Job drawing, mm, ordinate dimensions from the low corner. One solid piece. A direction names the side the tool comes from. Give positions to 0.01 mm unless a question says otherwise; leave off trailing zeros. Loops run counter-clockwise (first coordinate to the right, second up) from the corner with the lowest first, then second, coordinate; pieces in that order, holes last. Notation, with made-up numbers: (29, 28) -> (54, 28) arc R32 cw to (54, 60) -> close; hole circle Ø8 at (27.25, 3). An arc over 180 degrees is marked (long way). Answer as a JSON object with one key per item and string values. Group by question number.
Q1. Wall check: probe 1 along Z at (x, y) = (4, 3.3); probe 2 along X at (y, z) = (3.3, 3.5); probe 3 along Y at (x, z) = (6.5, 0.75) (3 decimals). Give the ranges that are in metal, low to high. Write a range as from..to.
Q2. Band-saw the part on C-C, the plane x = 1.25. Write the cut outline in (y, z) (3 decimals).
Q3. Drop flat-ended pins along their axis: pin 1 (1.2 mm diameter, centred on x = 3.5, z = 3.5, fed in from -Y); pin 2 (2 mm diameter, centred on y = 1, z = 4.5, fed in from +X). Give the stop position or say it passes through.
Q4. Band-saw the part on D-D, the plane z = 1. Write the cut outline in (x, y) (3 decimals).
Q5. Tool access for the marked faces 4, 5 and 6: list every direction of +Z, -Z, +X, -X, +Y, -Y with a clear straight run to the whole face (end or side of a thin tool).
Q6. Two-plate mould, pull along Z, no slides. Class the marked faces 1, 2 and 3: pulls with the +Z half, pulls with the -Z half, needs draft (parallel to the pull), parting line crosses it, or undercut.
Q7. Band-saw the part on B-B, the plane y = 2.5. Write the cut outline in (x, z).
Q8. Band-saw the part on A-A, the plane z = 4. Write the cut outline in (x, y) (1 decimal).
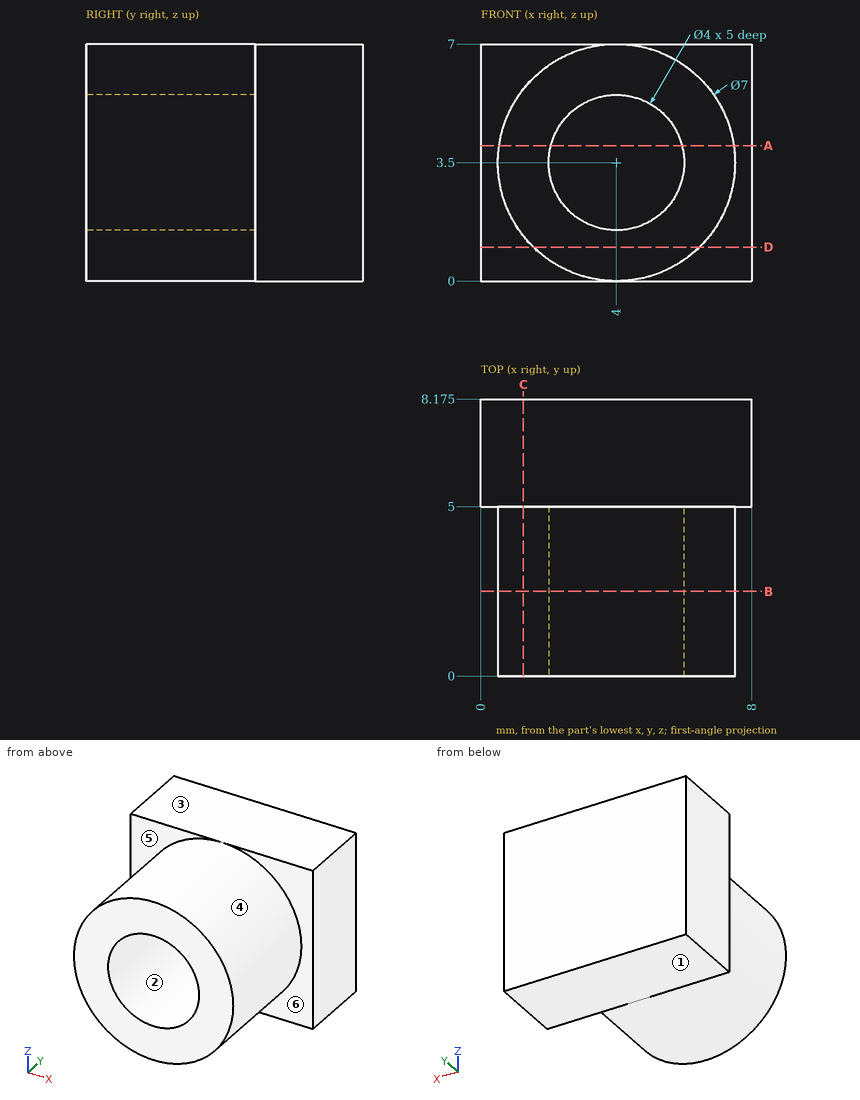
Worked answers:
{
 "1": {"probe 1": "0..1.5, 5.5..7", "probe 2": "0.5..2, 6..7.5", "probe 3": "5..8.175"},
 "2": {"outline": "(0, 1.335) -> (5, 1.335) -> (5, 0) -> (8.175, 0) -> (8.175, 7) -> (5, 7) -> (5, 5.665) -> (0, 5.665) -> close"},
 "3": {"pin 1": "y = 5", "pin 2": "x = 7.5"},
 "4": {"outline": "(0, 5) -> (1.551, 5) -> (1.551, 0) -> (6.449, 0) -> (6.449, 5) -> (8, 5) -> (8, 8.175) -> (0, 8.175) -> close"},
 "5": {"face 4": "-Y", "face 5": "-X, -Y", "face 6": "+X, -Y"},
 "6": {"face 1": "pulls with the -Z half", "face 2": "undercut", "face 3": "pulls with the +Z half"},
 "7": {"outline": "circle Ø7 at (4, 3.5); hole circle Ø4 at (4, 3.5)"},
 "8": {"outline": "(0, 5) -> (0.5, 5) -> (0.5, 0) -> (2.1, 0) -> (2.1, 5) -> (5.9, 5) -> (5.9, 0) -> (7.5, 0) -> (7.5, 5) -> (8, 5) -> (8, 8.2) -> (0, 8.2) -> close"}
}
